Input: part model. Units: mm. Frame: model coordinates. A direction names the side the tool comes from. Give positions to 0.01 mm unless a question says otherwise; leave off trailing zeros. Write each loop counter-clockwise with the first axis right and the second up, starting at its lowest first coordinate (ties: lowest second). Pieces come first, ordered by that corner, then holes. Notation, with made-up numbers: (36, -29) - (76, -29) arc R23 cw to (76, -2) - close; hole circle Ø5 at (27, 17.5). An arc over 180 degrees is marked (long way). Use a Markdown table: item, result. Add a question column.
1. Section query D-D, the plane x = 0. Return loops of the section in (y, z), plus the area to 3 significant figures.
2. Section query B-B, the plane z = 7.25. Return loops of the section in (x, y).
3. Pin query (flat end, axial travel): pin 1 (8 mm diameter, centred on x = 5, y = 8.5, fed in from -Z); pin 2 (4 mm diameter, centred on y = -6.5, z = 6, fed in from +X); pin 3 (6 mm diameter, centred on x = -5, y = -0.5, fed in from +Z). Return the tip coordinate at first contact, or that it passes through.
4. Set-up query: faces 1 (the cylindrical face through (5.47, 9.27, -13.19)), 2 (the cylindrical face through (4.563, -0.112, 2.909)). Return all of +Z, -Z, +X, -X, +Y, -Y with unobstructed straight access to the full face (end or side cutting, diameter ignored); none if empty.
5. Section query A-A, the plane x = 10.75. Return loops of the section in (y, z).
6. Material intervals for probe 1 along Y at (x, z) = (-12.75, -4.25); probe 2 along Y at (x, z) = (5, -8); probe 3 along Y at (x, z) = (4.25, -1), sorted ascending.
7. Mould query, pull axis Y, two halves, no side actions, for faces 3 (the cylindrical face through (5.47, -9.23, -13.19)), 4 (the flat face through (6, 8, 0)). Classes: released by +Y, released by -Y, zero draft, split by the parting line, or undercut.
8. Section query C-C, the plane y = -1.75. Return loops of the section in (x, z).
```python
from build123d import *

# Parameters (mm, degrees)
SKETCH1_R           = 14.278677311
SKETCH1_R_2         = 5.411731441
BOSS_EXTRUDE1_DEPTH = 10.5
SKETCH1_3_R         = 14.278677311
SKETCH1_3_R_2       = 5.411731441
CUT_EXTRUDE1_DEPTH  = 8
DOME1_FACE_RADIUS   = 14.278677311
DOME1_HEIGHT        = 2
DOME2_FACE_RADIUS   = 14.278677311
DOME2_HEIGHT        = 2


with BuildPart() as part:
    # Sketch1 → Boss-Extrude1 (new, symmetric)
    with BuildSketch(Plane(origin=(0, 0, 0), x_dir=(1, 0, 0), z_dir=(0, 1, 0))):
        with Locations(Location((0, 0, 0), (0, 0, 90))):
            Circle(SKETCH1_R)
        Circle(SKETCH1_R_2, mode=Mode.SUBTRACT)
        Circle(SKETCH1_R_2)
    extrude(amount=BOSS_EXTRUDE1_DEPTH, both=True)

    # Sketch1<3> → Cut-Extrude1 (cut, symmetric)
    with BuildSketch(Plane(origin=(0, 0, 0), x_dir=(1, 0, 0), z_dir=(0, 1, 0))):
        with Locations(Location((0, 0, 0), (0, 0, 90))):
            Circle(SKETCH1_3_R)
        with Locations(Location((0, 0, 0), (0, 0, 270))):
            Circle(SKETCH1_3_R_2, mode=Mode.SUBTRACT)
    extrude(amount=CUT_EXTRUDE1_DEPTH, both=True, mode=Mode.SUBTRACT)

    # Dome1: a dome of height H over a round flat face of radius A is a cap of a sphere of radius (A * A + H * H) / (2 * H)
    dome1_r = (DOME1_FACE_RADIUS * DOME1_FACE_RADIUS + DOME1_HEIGHT * DOME1_HEIGHT) / (2 * DOME1_HEIGHT)
    dome1_base = Plane((0, -10.5, 0), z_dir=(0, -1, 0))
    with Locations(dome1_base.offset(DOME1_HEIGHT - dome1_r)):
        dome1_ball = Sphere(dome1_r, mode=Mode.PRIVATE)
    add(split(dome1_ball, bisect_by=dome1_base, keep=Keep.TOP, mode=Mode.PRIVATE))

    # Dome2: a dome of height H over a round flat face of radius A is a cap of a sphere of radius (A * A + H * H) / (2 * H)
    dome2_r = (DOME2_FACE_RADIUS * DOME2_FACE_RADIUS + DOME2_HEIGHT * DOME2_HEIGHT) / (2 * DOME2_HEIGHT)
    dome2_base = Plane((0, 10.5, 0), z_dir=(0, 1, 0))
    with Locations(dome2_base.offset(DOME2_HEIGHT - dome2_r)):
        dome2_ball = Sphere(dome2_r, mode=Mode.PRIVATE)
    add(split(dome2_ball, bisect_by=dome2_base, keep=Keep.TOP, mode=Mode.PRIVATE))


solid = part.part
```
Result sheet:
| question | item | result |
|---|---|---|
| 1 | outline | (-10.5, -14.28) - (-8, -14.28) - (-8, -5.41) - (8, -5.41) - (8, -14.28) - (10.5, -14.28) arc R51.97 ccw to (10.5, 14.28) - (8, 14.28) - (8, 5.41) - (-8, 5.41) - (-8, 14.28) - (-10.5, 14.28) arc R51.97 ccw to start |
| 1 | area | 392 mm² |
| 2 | outline | (-12.3, -10.5) arc R51.46 ccw to (12.3, -10.5) - (12.3, -8) - (-12.3, -8) - close; (-12.3, 8) - (12.3, 8) - (12.3, 10.5) arc R51.46 ccw to (-12.3, 10.5) - close |
| 3 | pin 1 | stops at z = -14.24 |
| 3 | pin 2 | stops at x = 13.49 |
| 3 | pin 3 | stops at z = 5.03 |
| 4 | face 1 | +Y, -Y |
| 4 | face 2 | none |
| 5 | outline | (-10.5, -9.4) - (-8, -9.4) - (-8, 9.4) - (-10.5, 9.4) arc R50.85 ccw to start; (8, -9.4) - (10.5, -9.4) arc R50.85 ccw to (10.5, 9.4) - (8, 9.4) - close |
| 6 | probe 1 | y = -10.73 to -8, 8 to 10.73 |
| 6 | probe 2 | y = -11.64 to -8, 8 to 11.64 |
| 6 | probe 3 | y = -12.32 to 12.32 |
| 7 | face 3 | zero draft |
| 7 | face 4 | undercut |
| 8 | outline | circle Ø10.82 at (0, 0) |
